from build123d import *

# Parameters (mm, degrees)
SKETCH_W  = 27.8
SKETCH_H  = 15.9
SKETCH_R  = 1.7
PAD_DEPTH = 3
FILLET_R  = 2


with BuildPart() as part:
    # Sketch → Pad (new body)
    with BuildSketch(Plane.XY):
        Rectangle(SKETCH_W, SKETCH_H)
        with Locations((-11.1, -5.15)):
            Circle(SKETCH_R, mode=Mode.SUBTRACT)
        with Locations((11.1, 5.15)):
            Circle(SKETCH_R, mode=Mode.SUBTRACT)
    extrude(amount=PAD_DEPTH)

    # Fillet
    fillet_edges = [part.edges().sort_by_distance(p)[0] for p in [
        (13.9, -7.95, 1.5),
        (13.9, 7.95, 1.5),
        (-13.9, -7.95, 1.5),
        (-13.9, 7.95, 1.5),
    ]]
    fillet(fillet_edges, radius=FILLET_R)


solid = part.part
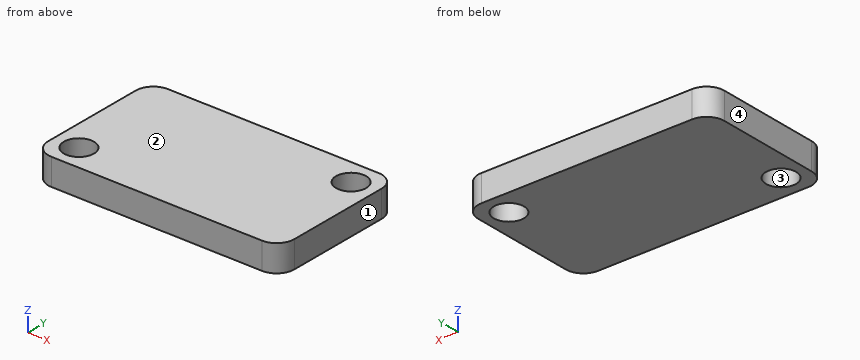
Verification items for the finished model (mm, model axes). Face numbers are marked on the shaded views. Round coordinates to 2 decimals unless told otherwise and drop trailing zeros. Loops run counter-clockwise (first coordinate to the right, second up) from the corner with the lowest first, then second, coordinate; pieces in that order, holes last. Notation, with made-up numbers: (-1.75, -26.75) - (19.25, -26.75) arc R24 ccw to (19.25, 3.25) - close; hole circle Ø10 at (50, 83.5). An arc over 180 degrees is marked (long way). Answer in a Markdown table with one row per item. Add a question column.
Q1. Release check for a two-part mould opening along X. For the marked faces 1, 2, 3 and 4 record: pulls with the +X half, pulls with the -X half, needs draft (parallel to the pull), parting line crosses it, or undercut.
Q2. Material ranges on line 1 (Y direction, x = -11.1, z = 1.55); line 2 (Y direction, x = 11.1, z = 1); line 3 (X direction, y = -4, z = 1.8), recorded low to high.
Q3. Gauge pin test, flat ends, axial feed: pin 1 (6 mm diameter, centred on x = -8, y = 4, fed in from -Z); pin 2 (2 mm diameter, centred on x = -11.1, y = -5.15, fed in from -Z). Record the tip position at first contact, or that the pin passes through.
Q4. Section check B-B on y = 5.15. Enter the section's corners in (x, z), plus the area to 3 significant figures.
Q5. Section check C-C on x = 11.1. Enter the section's corners in (y, z).
Q6. Section check A-A on z = 2. Enter the section's corners in (x, y), plus the area to 3 significant figures.
Found:
| question | item | result |
|---|---|---|
| 1 | face 1 | pulls with the +X half |
| 1 | face 2 | needs draft |
| 1 | face 3 | undercut |
| 1 | face 4 | pulls with the -X half |
| 2 | line 1 | y = -7.95 to -6.85, -3.45 to 7.95 |
| 2 | line 2 | y = -7.95 to 3.45, 6.85 to 7.95 |
| 2 | line 3 | x = -13.9 to -12.35, -9.85 to 13.9 |
| 3 | pin 1 | stops at z = 0 |
| 3 | pin 2 | passes through |
| 4 | outline | (-13.9, 0) - (9.4, 0) - (9.4, 3) - (-13.9, 3) - close; (12.8, 0) - (13.9, 0) - (13.9, 3) - (12.8, 3) - close |
| 4 | area | 73.2 mm² |
| 5 | outline | (-7.95, 0) - (3.45, 0) - (3.45, 3) - (-7.95, 3) - close; (6.85, 0) - (7.95, 0) - (7.95, 3) - (6.85, 3) - close |
| 6 | outline | (-13.9, -5.95) arc R2 ccw to (-11.9, -7.95) - (11.9, -7.95) arc R2 ccw to (13.9, -5.95) - (13.9, 5.95) arc R2 ccw to (11.9, 7.95) - (-11.9, 7.95) arc R2 ccw to (-13.9, 5.95) - close; hole circle Ø3.4 at (-11.1, -5.15); hole circle Ø3.4 at (11.1, 5.15) |
| 6 | area | 420 mm² |
